```python
from build123d import *

# Parameters (mm, degrees)
F0_W     = 300
F0_H     = 285
F1_DEPTH = 18
F2_R     = 5
F3_DEPTH = 18.001
F4_SIZE  = 10


with BuildPart() as f1:
    # F0 (on Right) → F1 (new body)
    with BuildSketch(Plane.YZ):
        with Locations((150, 142.5)):
            Rectangle(F0_W, F0_H)
    extrude(amount=F1_DEPTH)

    # F2 (on face) → F3 (cut, through all)
    with BuildSketch(Plane.YZ.offset(18)):
        with Locations((45, 255)):
            Circle(F2_R)
        with Locations((75, 255)):
            Circle(F2_R)
        with Locations((105, 255)):
            Circle(F2_R)
        with BuildLine():
            Line((80, 125), (50, 125))
            ThreePointArc((50, 125), (45, 120), (50, 115))
            Line((50, 115), (80, 115))
            Line((80, 115), (110, 115))
            ThreePointArc((110, 115), (115, 120), (110, 125))
            Line((110, 125), (80, 125))
        make_face()
        with BuildLine():
            ThreePointArc((50, 185), (45, 180), (50, 175))
            Line((50, 175), (80, 175))
            Line((80, 175), (110, 175))
            ThreePointArc((110, 175), (115, 180), (110, 185))
            Line((110, 185), (80, 185))
            Line((80, 185), (50, 185))
        make_face()
        with BuildLine():
            ThreePointArc((190, 185), (185, 180), (190, 175))
            Line((190, 175), (220, 175))
            Line((220, 175), (250, 175))
            ThreePointArc((250, 175), (255, 180), (250, 185))
            Line((250, 185), (220, 185))
            Line((220, 185), (190, 185))
        make_face()
        with BuildLine():
            ThreePointArc((190, 125), (185, 120), (190, 115))
            Line((190, 115), (220, 115))
            Line((220, 115), (250, 115))
            ThreePointArc((250, 115), (255, 120), (250, 125))
            Line((250, 125), (220, 125))
            Line((220, 125), (190, 125))
        make_face()
    extrude(amount=-F3_DEPTH, mode=Mode.SUBTRACT)

    # F4
    f4_edges = [f1.edges().sort_by_distance(p)[0] for p in [
        (9, 0, 285),
        (9, 300, 285),
    ]]
    chamfer(f4_edges, length=F4_SIZE)


solid = f1.part
```
Input: part model. Units: mm. Frame: model coordinates. A direction names the side the tool comes from. Round coordinates to 2 decimals unless told otherwise and drop trailing zeros. Write each loop counter-clockwise with the first axis right and the second up, starting at its lowest first coordinate (ties: lowest second). Pieces come first, ordered by that corner, then holes. Notation, with made-up numbers: (49.5, 55) - (89.5, 55) arc R4 cw to (89.5, 61) - close; hole circle Ø3 at (43, 49.25). An arc over 180 degrees is marked (long way). Write item = value, one per line.
(1) Material intervals for probe 1 along Z at (x, y) = (9.25, 75); probe 2 along Z at (x, y) = (7, 110.5), sorted ascending.
Geometry check:
probe_1 = 0 to 115, 125 to 175, 185 to 250, 260 to 285
probe_2 = 0 to 115.03, 124.97 to 175.03, 184.97 to 285
(2) Section query A-A on y = 75. Output: boundary loops of the cut face in (x, z), then the cut area to 3 significant figures.
Geometry check:
outline = (0, 0) - (18, 0) - (18, 115) - (0, 115) - close; (0, 125) - (18, 125) - (18, 175) - (0, 175) - close; (0, 185) - (18, 185) - (18, 250) - (0, 250) - close; (0, 260) - (18, 260) - (18, 285) - (0, 285) - close
area = 4,590 mm^2
(3) Access query for faces 4 (the flat face through (9, 80, 175)), 5 (the flat face through (9, 5, 280)). Directions: +Z, -Z, +X, -X, +Y, -Y. A direction counts if a zero-diameter tool reaches every point of the face in a straight line with its end or side. Return the directions, or none.
Geometry check:
face_4 = +X, -X
face_5 = +Z, +X, -X, -Y
(4) Contact query for a flat-ended pin moving along its axis: pin 1 Ø13 at (y, z) = (45, 255) entering from +X. Output: stop coordinate, or through.
Geometry check:
pin_1 = 18
(5) Section query B-B on x = 14.5. Output: boundary loops of the cut face in (y, z).
Geometry check:
outline = (0, 0) - (300, 0) - (300, 275) - (290, 285) - (10, 285) - (0, 275) - close; hole circle Ø10 at (45, 255); hole (50, 115) - (110, 115) arc R5 ccw to (110, 125) - (50, 125) arc R5 ccw to start; hole (50, 175) - (110, 175) arc R5 ccw to (110, 185) - (50, 185) arc R5 ccw to start; hole circle Ø10 at (75, 255); hole circle Ø10 at (105, 255); hole (190, 115) - (250, 115) arc R5 ccw to (250, 125) - (190, 125) arc R5 ccw to start; hole (190, 175) - (250, 175) arc R5 ccw to (250, 185) - (190, 185) arc R5 ccw to start
(6) Pull-direction query (Z, two-part tool) for faces 1 (the flat face through (9, 148, 285)), 2 (the flat face through (9, 0, 136)), 3 (the cylindrical face through (9, 78, 259)); classes: +Z half, -Z half, draft (parallel to the pull), parting line (faces both ways), or undercut.
Geometry check:
face_1 = +Z half
face_2 = draft
face_3 = undercut
(7) Section query C-C on z = 120. Output: boundary loops of the cut face in (x, y), then the cut area to 3 significant figures.
Geometry check:
outline = (0, 0) - (18, 0) - (18, 45) - (0, 45) - close; (0, 115) - (18, 115) - (18, 185) - (0, 185) - close; (0, 255) - (18, 255) - (18, 300) - (0, 300) - close
area = 2,880 mm^2
